from build123d import *

# Parameters (mm, degrees)
SKETCH1_R               = 40
BOSS_EXTRUDE1_DEPTH     = 37.5
SKETCH3_R               = 7.5
CUT_EXTRUDE2_DEPTH      = 41
CUT_EXTRUDE2_DEPTH_BACK = 41
REVOLVE1_ANGLE          = 180
SKETCH2_R               = 35
CUT_EXTRUDE3_DEPTH      = 90


with BuildPart() as part:
    # Sketch1 → Boss-Extrude1 (new body, symmetric)
    with BuildSketch(Plane.XY):
        Circle(SKETCH1_R)
    extrude(amount=BOSS_EXTRUDE1_DEPTH, both=True)

    # Sketch3 → Cut-Extrude2 (cut, two sides)
    with BuildSketch(Plane(origin=(0, 0, 0), x_dir=(0, 0, -1), z_dir=(1, 0, 0))) as cut_extrude2_sk:
        with Locations((17.5, 0)):
            Circle(SKETCH3_R)
    extrude(amount=CUT_EXTRUDE2_DEPTH, mode=Mode.SUBTRACT)
    extrude(cut_extrude2_sk.sketch, amount=-CUT_EXTRUDE2_DEPTH_BACK, mode=Mode.SUBTRACT)

    # Sketch7 → Revolve1 (revolve)
    with BuildSketch(Plane(origin=(0, 0, -37.5), x_dir=(-1, 0, 0), z_dir=(0, 0, -1))):
        with BuildLine():
            Line((0, 40), (0, -40))
            ThreePointArc((0, -40), (-40, 0), (0, 40))
        make_face()
    revolve(axis=Axis((0, 40, -37.5), (0, 1, 0)), revolution_arc=REVOLVE1_ANGLE)

    # Sketch2 → Cut-Extrude3 (cut)
    with BuildSketch(Plane.XY.offset(37.5)):
        Circle(SKETCH2_R)
    extrude(amount=-CUT_EXTRUDE3_DEPTH, mode=Mode.SUBTRACT)


solid = part.part
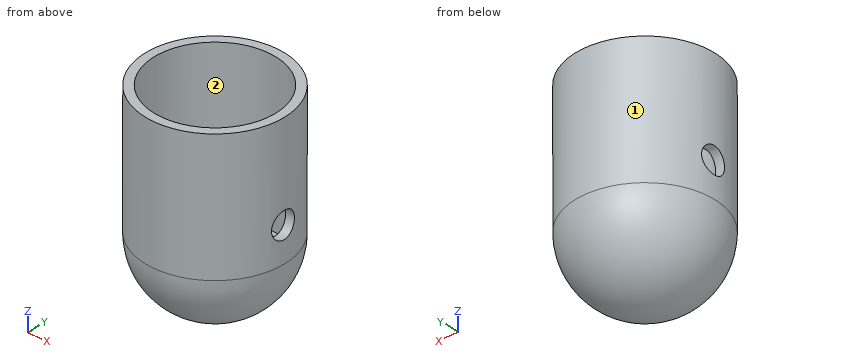
Could you check a few things on this model? Use its own coordinates, in mm. Face numbers are marked on the shaded views. Give positions to 0.01 mm unless a question says otherwise; leave off trailing zeros. Order: outer loops, then holes, each group sorted by start corner. A loop starts at its lowest first (then second) coordinate and runs counter-clockwise, first axis right, second up. Notation, with made-up numbers: (42, 57) -> (60, 57) arc R34 ccw to (60, 89) -> close; hole circle Ø2 at (80, 43). An arc over 180 degrees is marked (long way). Return JSON: item names as keys, results as strings.
1. For pin 1 Ø1 at (y, z) = (-21.5, 15.5) entering from -X; pin 2 Ø1.5 at (x, y) = (-1, -17) entering from +Z; pin 3 Ø1 at (y, z) = (19, -47) entering from -X, each with a flat end and sliding along its axis, tell me the tip position at first contact or that it passes through.
Answer list:
{"pin 1": "stops at x = -34.04", "pin 2": "stops at z = -52.5", "pin 3": "stops at x = -34.2"}
2. Imagine slicing it at C-C on y = -32. List the corners of the cut face in (x, z) for me, then the cut area to 3 significant figures.
Answer list:
{"outline": "(-24, -37.5) arc R24 ccw to (24, -37.5) -> (24, 37.5) -> (14.18, 37.5) -> (14.18, -52.5) -> (-14.18, -52.5) -> (-14.18, 37.5) -> (-24, 37.5) -> close", "area": "1,950 mm2"}
3. I need wall thicknesses on line 1 (X direction, y = 0, z = 19); line 2 (X direction, y = -23.5, z = 21); line 3 (Y direction, x = 20, z = -48.5). Which ranges of each line are inside material? Lowest first, please. Write a range as from..to.
Answer list:
{"line 1": "x = -40..-35, 35..40", "line 2": "x = -32.37..-25.94, 25.94..32.37", "line 3": "y = -32.85..-28.72, 28.72..32.85"}
4. Imagine slicing it at D-D on z = -17.5. List the corners of the cut face in (x, y) for me, then the cut area to 3 significant figures.
Answer list:
{"outline": "(-39.29, -7.5) arc R40 ccw to (39.29, -7.5) -> (34.19, -7.5) arc R35 cw to (-34.19, -7.5) -> close; (-39.29, 7.5) -> (-34.19, 7.5) arc R35 cw to (34.19, 7.5) -> (39.29, 7.5) arc R40 ccw to start", "area": "1,030 mm2"}
5. Imagine slicing it at A-A on z = 19. List the corners of the cut face in (x, y) for me.
Answer list:
{"outline": "circle Ø80 at (0, 0); hole circle Ø70 at (0, 0)"}
6. Imagine slicing it at B-B on x = 0. List the corners of the cut face in (y, z) for me.
Answer list:
{"outline": "(-40, -37.5) arc R40 ccw to (40, -37.5) -> (40, 37.5) -> (35, 37.5) -> (35, -52.5) -> (-35, -52.5) -> (-35, 37.5) -> (-40, 37.5) -> close"}
7. Thinking about a two-plate mould opening in X: for the marked faces 1 and 2, which applies, pulls with the +X half, pulls with the -X half, needs draft (parallel to the pull), parting line crosses it, or undercut?
Answer list:
{"face 1": "parting line crosses it", "face 2": "undercut"}
